Geometry: final body of the model. Coordinates: model frame, mm. A direction names the side the tool comes from. Coordinates: 2 decimals unless noted, no trailing zeros. Order: outer loops, then holes, each group sorted by start corner. A loop starts at its lowest first (then second) coordinate and runs counter-clockwise, first axis right, second up. Notation, with made-up numbers: M 11.25,-0.5 L 39.25,-0.5 A5 cw 39.25,3.5 Z; hole C -37.75,64 d2. An arc over 180 degrees is marked long. Use CSV: the item, a comma, the result in double quotes. Start each with the question number.
1. First-contact query: P1, Ø10, axis at x = -125, y = -14, coming from the +Z side; P2, Ø6, axis at y = -28, z = 12, coming from the +X side; P3, Ø5, axis at y = -19.5, z = -6, coming from the -X side. Flat tips, straight axial feed; report the tip coordinate or a pass-through.
2. Section query B-B on x = 81.5. Return the cut outline in (y, z), and give its area (4 significant figures).
3. Material intervals for line 1 (Y direction, x = -31.5, z = 2); line 2 (Z direction, x = 185, y = -34.95); line 3 (X direction, y = 9.5, z = 2.5), sorted ascending.
4. Section query A-A on y = 13. Return the cut outline in (x, z).
5. Pull-direction query (X, two-part tool) for faces 5 (the flat face through (-195, 0, 13)), 6 (the flat face through (3, -35.5, 11)), 7 (the cylindrical face through (171, -23.5, 0.5)); classes: pulls with the +X half, pulls with the -X half, needs draft (parallel to the pull), parting line crosses it, or undercut.
6. Set-up query: faces 1 (the flat face through (1, 35.5, 6)), 2 (the flat face through (-3, 0, 0)), 3 (the flat face through (-2, -34.5, 9)), 4 (the flat face through (-157.5, -17, 8)). Return all of +Z, -Z, +X, -X, +Y, -Y with unobstructed straight access to the full face (end or side cutting, diameter ignored); none if empty.
from build123d import *

# Parameters (mm, degrees)
CROQUIS1_W               = 390
CROQUIS1_H               = 71
SALIENTE_EXTRUIR1_DEPTH  = 1
CROQUIS3_W               = 356.15
CROQUIS3_H               = 1
SALIENTE_EXTRUIR3_DEPTH  = 10
CROQUIS4_W               = 356.15
CROQUIS4_H               = 1
SALIENTE_EXTRUIR4_DEPTH  = 3.5
CROQUIS5_W               = 30
CROQUIS5_H               = 1
SALIENTE_EXTRUIR5_DEPTH  = 13.5
CROQUIS6_W               = 0.5
CROQUIS6_H               = 70
SALIENTE_EXTRUIR6_DEPTH  = 26
CROQUIS7_W               = 390
CROQUIS7_H               = 1
SALIENTE_EXTRUIR7_DEPTH  = 18
CROQUIS8_W               = 390
CROQUIS8_H               = 1
SALIENTE_EXTRUIR8_DEPTH  = 4
CORTAR_EXTRUIR1_REACH    = 202.391
CROQUIS11_W              = 36
CROQUIS11_H              = 10
CROQUIS12_W              = 1
CROQUIS12_H              = 10
SALIENTE_EXTRUIR11_DEPTH = 15
REDONDEO1_R              = 3
CROQUIS13_R              = 2
SALIENTE_EXTRUIR12_DEPTH = 1
CORTAR_EXTRUIR2_REACH    = 395.039
CROQUIS14_R              = 1.75
CROQUIS16_R              = 5
CROQUIS16_R_2            = 1.3
CORTAR_EXTRUIR4_DEPTH    = 1
CROQUIS25_R              = 1.25
CROQUIS25_R_2            = 2.5
CORTAR_EXTRUIR5_DEPTH    = 1
CROQUIS30_W              = 1
CROQUIS30_H              = 71
SALIENTE_EXTRUIR15_DEPTH = 15
CROQUIS31_R              = 1.75
CORTAR_EXTRUIR12_DEPTH   = 1


with BuildPart() as part:
    # Croquis1 → Saliente-Extruir1 (new body)
    with BuildSketch(Plane.XY):
        Rectangle(CROQUIS1_W, CROQUIS1_H)
    extrude(amount=SALIENTE_EXTRUIR1_DEPTH)

    # Croquis3 → Saliente-Extruir3 (add)
    with BuildSketch(Plane.XY.offset(1)):
        with Locations((13.075, 35)):
            Rectangle(CROQUIS3_W, CROQUIS3_H)
    extrude(amount=SALIENTE_EXTRUIR3_DEPTH)

    # Croquis4 → Saliente-Extruir4 (add)
    with BuildSketch(Plane.XZ.offset(-34.5)):
        with Locations((13.075, 10.5)):
            Rectangle(CROQUIS4_W, CROQUIS4_H)
    extrude(amount=SALIENTE_EXTRUIR4_DEPTH)

    # Croquis5 → Saliente-Extruir5 (add)
    with BuildSketch(Plane.XY.offset(1)):
        with Locations((-180, 35)):
            Rectangle(CROQUIS5_W, CROQUIS5_H)
    extrude(amount=SALIENTE_EXTRUIR5_DEPTH)

    # Croquis6 → Saliente-Extruir6 (add)
    with BuildSketch(Plane.XY.offset(1)):
        with Locations((-194.75, -0.5)):
            Rectangle(CROQUIS6_W, CROQUIS6_H)
    extrude(amount=SALIENTE_EXTRUIR6_DEPTH)

    # Croquis7 → Saliente-Extruir7 (add)
    with BuildSketch(Plane.XY.offset(1)):
        with Locations((0.5, -35)):
            Rectangle(CROQUIS7_W, CROQUIS7_H)
    extrude(amount=SALIENTE_EXTRUIR7_DEPTH)

    # Croquis8 → Saliente-Extruir8 (add)
    with BuildSketch(Plane(origin=(0, -34.5, 0), x_dir=(1, 0, 0), z_dir=(0, 1, 0))):
        with Locations((0.5, -18.5)):
            Rectangle(CROQUIS8_W, CROQUIS8_H)
    extrude(amount=SALIENTE_EXTRUIR8_DEPTH)

    # Croquis11 → Cortar-Extruir1 (cut, up to next)
    with BuildSketch(Plane.XY.offset(1), mode=Mode.PRIVATE) as cortar_extruir1_sk1:
        with Locations((-176.5, -16.5)):
            Rectangle(CROQUIS11_W, CROQUIS11_H)
    cortar_extruir1_tool1 = extrude(cortar_extruir1_sk1.sketch, amount=-CORTAR_EXTRUIR1_REACH, mode=Mode.PRIVATE) & part.part
    add(cortar_extruir1_tool1.solids().sort_by_distance((-176.5, -16.5, 1))[0], mode=Mode.SUBTRACT)

    # Croquis12 → Saliente-Extruir11 (add)
    with BuildSketch(Plane.XY.offset(1)):
        with Locations((-158, -16.5)):
            Rectangle(CROQUIS12_W, CROQUIS12_H)
    extrude(amount=SALIENTE_EXTRUIR11_DEPTH)

    # Redondeo1
    redondeo1_edges = [part.edges().sort_by_distance(p)[0] for p in [
        (-158, -21.5, 16),
        (-158, -11.5, 16),
    ]]
    fillet(redondeo1_edges, radius=REDONDEO1_R)

    # Croquis13 → Saliente-Extruir12 (add)
    with BuildSketch(Plane.ZY.offset(158.5)):
        with Locations(Location((10.5, -16.5, 0), (0, 0, 180))):
            Circle(CROQUIS13_R)
    extrude(amount=SALIENTE_EXTRUIR12_DEPTH)

    # Croquis14 → Cortar-Extruir2 (cut, up to next)
    with BuildSketch(Plane.ZY.offset(195), mode=Mode.PRIVATE) as cortar_extruir2_sk1:
        with Locations((5.81, 30.25)):
            Circle(CROQUIS14_R)
    cortar_extruir2_tool1 = extrude(cortar_extruir2_sk1.sketch, amount=-CORTAR_EXTRUIR2_REACH, mode=Mode.PRIVATE) & part.part
    add(cortar_extruir2_tool1.solids().sort_by_distance((-195, 30.25, 5.81))[0], mode=Mode.SUBTRACT)

    # Croquis16 → Cortar-Extruir4 (cut)
    with BuildSketch(Plane.XY.offset(1)):
        with Locations((175, -20.5)):
            Circle(CROQUIS16_R)
        with Locations((184.526279442, -26)):
            Circle(CROQUIS16_R_2)
        with Locations((165.473720558, -15)):
            Circle(CROQUIS16_R_2)
    extrude(amount=-CORTAR_EXTRUIR4_DEPTH, mode=Mode.SUBTRACT)

    # Croquis25 → Cortar-Extruir5 (cut)
    with BuildSketch(Plane.XZ.offset(35.5)):
        with Locations((-168.9, 4.78)):
            Circle(CROQUIS25_R)
        with Locations((-161.9, 4.78)):
            Circle(CROQUIS25_R_2)
        with Locations((185, 6.05)):
            Circle(CROQUIS25_R)
        with Locations((178, 6.05)):
            Circle(CROQUIS25_R_2)
    extrude(amount=-CORTAR_EXTRUIR5_DEPTH, mode=Mode.SUBTRACT)

    # Croquis30 → Saliente-Extruir15 (add)
    with BuildSketch(Plane(origin=(0, 0, 0), x_dir=(-1, 0, 0), z_dir=(0, 0, -1))):
        with Locations((-194.5, 0)):
            Rectangle(CROQUIS30_W, CROQUIS30_H)
    extrude(amount=SALIENTE_EXTRUIR15_DEPTH)

    # Croquis31 → Cortar-Extruir12 (cut)
    with BuildSketch(Plane(origin=(195, 0, 0), x_dir=(0, 0, -1), z_dir=(1, 0, 0))):
        with Locations((5, 27.7)):
            Circle(CROQUIS31_R)
    extrude(amount=-CORTAR_EXTRUIR12_DEPTH, mode=Mode.SUBTRACT)


solid = part.part
Results list:
1,P1,"stops at z = 1"
1,P2,"stops at x = -194.5"
1,P3,"stops at x = 194"
2,outline,"M -35.5,0 L 35.5,0 L 35.5,11 L 31,11 L 31,10 L 34.5,10 L 34.5,1 L -34.5,1 L -34.5,18 L -30.5,18 L -30.5,19 L -35.5,19 Z"
2,area,"106.5 mm²"
3,line 1,"y = -35.5 to -34.5, 34.5 to 35.5"
3,line 2,"z = 0 to 4.8, 7.3 to 19"
3,line 3,"x = -195 to -194.5"
4,outline,"M -195,0 L 194,0 L 194,-15 L 195,-15 L 195,1 L -194.5,1 L -194.5,27 L -195,27 Z"
5,face 5,"pulls with the -X half"
5,face 6,"needs draft"
5,face 7,"undercut"
6,face 1,"+Z, -Z, +X, -X, +Y"
6,face 2,"-Z, -X, +Y, -Y"
6,face 3,"+X"
6,face 4,"+Z, +X"
